Drawing for the job (mm, zero at the part's lowest x, y, z). A direction names the side the tool comes from. Round coordinates to 2 decimals unless told otherwise and drop trailing zeros. Loops run counter-clockwise (first coordinate to the right, second up) from the corner with the lowest first, then second, coordinate; pieces in that order, holes last. Notation, with made-up numbers: (73.5, 38.25) - (128.5, 38.25) arc R12 ccw to (128.5, 49.25) - close; hole circle Ø9 at (72, 16). An arc over 180 degrees is marked (long way). Put each result on its own line as item: value.
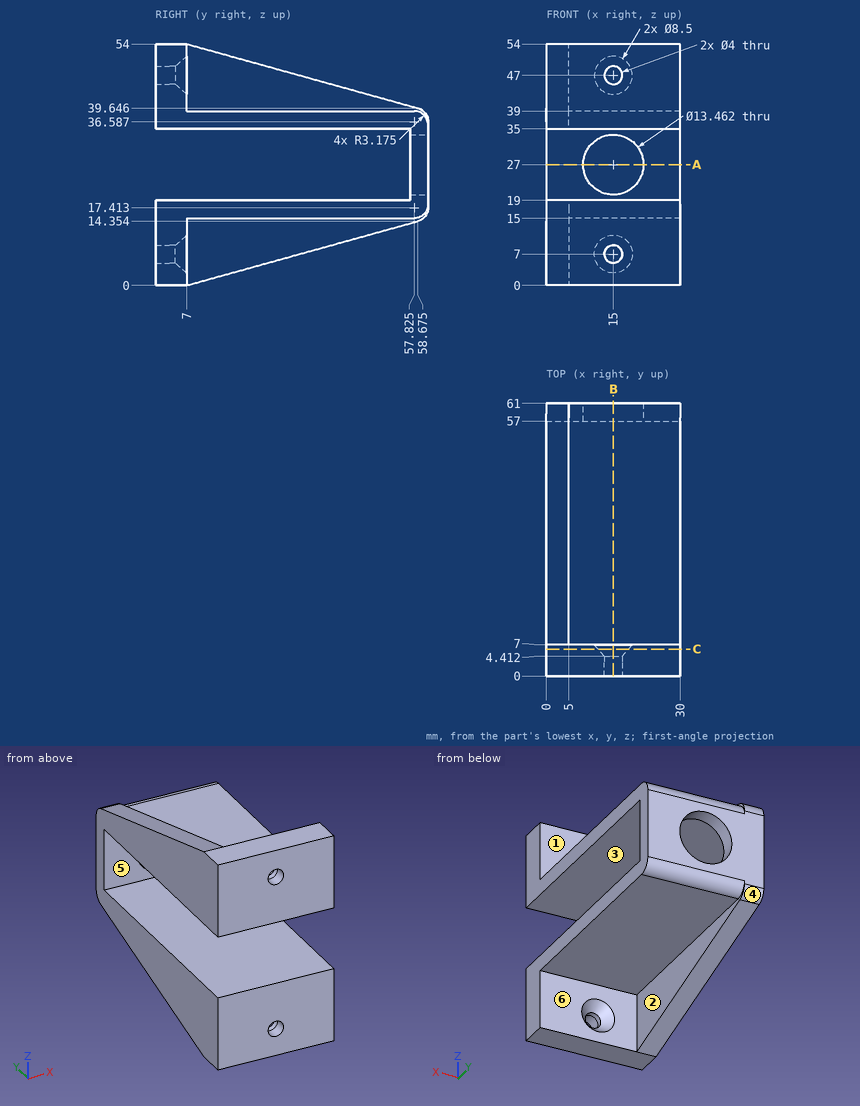
1. Band-saw the part on B-B (x = 15). Give the number of separate pieces and of enclosed holes in the cut face, plus the area to 3 significant figures.
A:
separate pieces: 4
enclosed holes: 0
area: 636 mm²
2. Band-saw the part on C-C (y = 6). List the corners of the cut face in (x, z), plus the area to 3 significant figures.
A:
outline: (0, 0) - (30, 0) - (30, 19) - (0, 19) - close; (0, 35) - (30, 35) - (30, 54) - (0, 54) - close; hole circle Ø6.76 at (15, 7); hole circle Ø6.76 at (15, 47)
area: 1,070 mm²
3. Two-plate mould, pull along Z, no slides. Class the marked faces 4, 5 and 6: pulls with the +Z half, pulls with the -Z half, needs draft (parallel to the pull), parting line crosses it, or undercut.
A:
face 4: pulls with the -Z half
face 5: undercut
face 6: needs draft
4. Probe line 1 along X through (y, z) = (3.9, 47); line 2 along Z through (x, y) = (20.25, 35); line 3 along X through (y, z) = (28, 40). List the from-to ranges inside material, lowest first. Write a range as [from, to].
A:
line 1: x = [0, 13], [17, 30]
line 2: z = [15, 19], [35, 39]
line 3: x = [0, 5]
5. Pin check, flat tips, straight feed: P1, Ø10, axis at x = 10.5, z = 8, coming from the +Y side; P2, Ø2, axis at x = 12, y = 16.5, coming from the +Z side; P3, Ø5, axis at x = 22, z = 24.5, coming from the -Y side. Stop position of each tip, or through.
A:
P1: stops at y = 7
P2: stops at z = 39
P3: stops at y = 57
6. Band-saw the part on A-A (z = 27). List the corners of the cut face in (x, y).
A:
outline: (0, 57) - (8.27, 57) - (8.27, 61) - (0, 61) - close; (21.73, 57) - (30, 57) - (30, 61) - (21.73, 61) - close
7. Tool access for the marked faces 1, 2 and 3: list every direction of +Z, -Z, +X, -X, +Y, -Y with a clear straight run to the whole face (end or side of a thin tool).
A:
face 1: +Z, +X, +Y
face 2: -Z, +X, +Y
face 3: +X, -X, -Y
